from build123d import *

# Parameters (mm, degrees)
F0_R           = 7.5
F1_DEPTH       = 20
F2_R           = 2.5
F3_DEPTH       = 20
F5_D           = 6
F5_DEPTH       = 20
F5_CBORE_D     = 10
F5_CBORE_DEPTH = 5
F5_TIP         = 1.8025818571


# Not quite as in the source:
# - a pattern or mirror of a feature is missing from the dataset's text; its kind, count and spacing are read off the source's solid


with BuildPart() as f1:
    # F0 (on Front) → F1 (new body)
    with BuildSketch(Plane.XZ):
        with BuildLine():
            Line((0, 42.5), (-30, 42.5))
            Line((-30, 42.5), (-30, -42.5))
            Line((-30, -42.5), (0, -42.5))
            Line((0, -42.5), (28.9472864716, -14.3343364017))
            ThreePointArc((28.9472864716, -14.3343364017), (35, 0), (28.9472864716, 14.3343364017))
            Line((28.9472864716, 14.3343364017), (0, 42.5))
        make_face()
        with Locations((15, 0)):
            Circle(F0_R, mode=Mode.SUBTRACT)
    extrude(amount=F1_DEPTH)

    # F2 (on face) → F3 (cut, through all)
    with BuildSketch(Plane.XZ.offset(20)):
        with Locations((-10, 32.5)):
            Circle(F2_R)
        with Locations((-10, -32.5)):
            Circle(F2_R)
    extrude(amount=-F3_DEPTH, mode=Mode.SUBTRACT)

    # F5
    with Locations(Plane.XZ.offset(20)):
        with Locations((-22, 34.5)):
            f5 = CounterBoreHole(F5_D / 2, F5_CBORE_D / 2, F5_CBORE_DEPTH, depth=F5_DEPTH)
            with Locations((0, 0, -(F5_DEPTH + F5_TIP / 2))):  # 118° drill point
                Cone(0, F5_D / 2, F5_TIP, mode=Mode.SUBTRACT)

    # F5_copies: F5 across plane
    add(f5.mirror(Plane(origin=(0, 0, 0), x_dir=(-1, 0, 0), z_dir=(0, 0, -1))), mode=Mode.SUBTRACT)


solid = f1.part
Here's how the part is built. I have some questions about the finished solid (model axes, mm). A direction names the side the tool comes from. Coordinates: 2 decimals unless noted, no trailing zeros. Write each loop counter-clockwise with the first axis right and the second up, starting at its lowest first coordinate (ties: lowest second). Pieces come first, ordered by that corner, then holes.
1) If we section it at B-B (y = -12.5): List the corners of the cut face in (x, z) for me.
Filled in:
outline: (-30, -42.5) - (0, -42.5) - (28.95, -14.33) arc R20 ccw to (28.95, 14.33) - (0, 42.5) - (-30, 42.5) - close; hole circle Ø6 at (-22, -34.5); hole circle Ø6 at (-22, 34.5); hole circle Ø5 at (-10, -32.5); hole circle Ø5 at (-10, 32.5); hole circle Ø15 at (15, 0)
2) Thinking about a two-plate mould opening in X: for faces 3 (the face through (-10, -10, -30)), 4 (the face through (-15, -10, 42.5)), 5 (the face through (-22.651, -17.535, 39.457)), 6 (the face through (14.676, -9.86, 28.22)), which applies, +X half, -X half, draft (parallel to the pull), parting line (faces both ways), or undercut?
Filled in:
face 3: undercut
face 4: draft
face 5: undercut
face 6: +X half
3) Which directions (+Z, -Z, +X, -X, +Y, -Y) give clear straight access to the entire face, cutting with the end or side of a thin tool? Please do faces 1 (the face through (-20, -15, 32)), 2 (the face through (-12, -10, 34)).
Filled in:
face 1: -Y
face 2: +Y, -Y
4) If I drill on line 1 (Z direction, x = -22, y = -10); line 2 (Z direction, x = -22, y = -16.7); line 3 (X direction, y = -4.5, z = -34.5), over which ranges is the centre line in solid material (lowest first)?
Filled in:
line 1: z = -42.5 to -37.5, -31.5 to 31.5, 37.5 to 42.5
line 2: z = -42.5 to -39.5, -29.5 to 29.5, 39.5 to 42.5
line 3: x = -30 to -25, -19 to -11.5, -8.5 to 8.22
5) If we section it at A-A (x = -10): List the corners of the cut face in (y, z) for me, plus the area to 3 significant figures.
Filled in:
outline: (-20, -42.5) - (0, -42.5) - (0, -35) - (-20, -35) - close; (-20, -30) - (0, -30) - (0, 30) - (-20, 30) - close; (-20, 35) - (0, 35) - (0, 42.5) - (-20, 42.5) - close
area: 1,500 mm2
6) I'm going to push flat-ended pins straight in: pin 1 (6 mm diameter, centred on x = 26.5, y = -3, fed in from +Z); pin 2 (6 mm diameter, centred on x = 27, y = -15.5, fed in from -Z); pin 3 (9.5 mm diameter, centred on x = -22, z = -34.5, fed in from +Y); pin 4 (3 mm diameter, centred on x = 20.5, y = -17.5, fed in from +Z). Where does each tip first touch, or does it pass through?
Filled in:
pin 1: stops at z = 19.63
pin 2: stops at z = -19.15
pin 3: stops at y = 0
pin 4: stops at z = 24.01
7) If we section it at D-D (x = 10): List the corners of the cut face in (y, z) for me.
Filled in:
outline: (-20, -32.77) - (0, -32.77) - (0, -5.59) - (-20, -5.59) - close; (-20, 5.59) - (0, 5.59) - (0, 32.77) - (-20, 32.77) - close
8) If we section it at C-C (z = 32.5): List the corners of the cut face in (x, y) for me, plus the area to 3 significant figures.
Filled in:
outline: (-30, -20) - (-26.58, -20) - (-26.58, -15) - (-24.24, -15) - (-24.24, 0) - (-30, 0) - close; (-19.76, -15) - (-17.42, -15) - (-17.42, -20) - (-12.5, -20) - (-12.5, 0) - (-19.76, 0) - close; (-7.5, -20) - (10.28, -20) - (10.28, 0) - (-7.5, 0) - close
area: 593 mm2
